from build123d import *

# Parameters (mm, degrees)
SKETCH1_R           = 29.5
BOSS_EXTRUDE1_DEPTH = 6
SKETCH2_R           = 15
BOSS_EXTRUDE2_DEPTH = 25
SKETCH3_R           = 3
CUT_EXTRUDE1_DEPTH  = 25
SKETCH4_R           = 2.5
CUT_EXTRUDE2_DEPTH  = 25


with BuildPart() as part:
    # Sketch1 → Boss-Extrude1 (new body)
    with BuildSketch(Plane(origin=(0, 0, 0), x_dir=(0, 0, -1), z_dir=(1, 0, 0))):
        Circle(SKETCH1_R)
    extrude(amount=BOSS_EXTRUDE1_DEPTH)

    # Sketch2 → Boss-Extrude2 (add)
    with BuildSketch(Plane(origin=(6, 0, 0), x_dir=(0, 0, -1), z_dir=(1, 0, 0))):
        Circle(SKETCH2_R)
    extrude(amount=BOSS_EXTRUDE2_DEPTH)

    # Sketch3 → Cut-Extrude1 (cut)
    with BuildSketch(Plane(origin=(31, 0, 0), x_dir=(0, 0, -1), z_dir=(1, 0, 0))):
        Circle(SKETCH3_R)
    extrude(amount=-CUT_EXTRUDE1_DEPTH, mode=Mode.SUBTRACT)

    # Sketch4 → Cut-Extrude2 (cut)
    with BuildSketch(Plane(origin=(6, 0, 0), x_dir=(0, 0, -1), z_dir=(1, 0, 0))):
        with Locations((0, 23.75)):
            Circle(SKETCH4_R)
        with Locations((20.56810334, 11.875)):
            Circle(SKETCH4_R)
        with Locations((20.56810334, -11.875)):
            Circle(SKETCH4_R)
        with Locations((0, -23.75)):
            Circle(SKETCH4_R)
        with Locations((-20.56810334, -11.875)):
            Circle(SKETCH4_R)
        with Locations((-20.56810334, 11.875)):
            Circle(SKETCH4_R)
    extrude(amount=-CUT_EXTRUDE2_DEPTH, mode=Mode.SUBTRACT)


solid = part.part
Geometry: final body of the model. Coordinates: model frame, mm. A direction names the side the tool comes from. Round coordinates to 2 decimals unless told otherwise and drop trailing zeros. Loops run counter-clockwise (first coordinate to the right, second up) from the corner with the lowest first, then second, coordinate; pieces in that order, holes last. Notation, with made-up numbers: M 8,10.5 L 29,10.5 A20 cw 29,19.5 Z; hole C -6.75,38 d2. An arc over 180 degrees is marked long. Put each result on its own line as item: value. Start each with the question number.
(1) Section query D-D (y = -23.75). Return loops of the section in (x, z), then the cut area to 3 significant figures.
(2) Section query B-B (y = 0). Return loops of the section in (x, z), then the cut area to 3 significant figures.
(3) Section query C-C (y = 13). Return loops of the section in (x, z).
(4) Set-up query: faces 5 (the face through (6, 0, 0)), 6 (the face through (3.04, 26.23, 0.33)). Return all of +Z, -Z, +X, -X, +Y, -Y with unobstructed straight access to the full face (end or side cutting, diameter ignored); none if empty.
(5) Contact query for flat-ended pins moving along their axis: pin 1 Ø5 at (x, z) = (26.5, -4) entering from -Y; pin 2 Ø5 at (x, z) = (25, 2.5) entering from -Y; pin 3 Ø8 at (y, z) = (11.88, -20.57) entering from +X. Output: stop coordinate, or through.
(6) Draft query along Y for faces 1 (the face through (0, 0, 0)), 2 (the face through (18.325, 0.66, 14.985)), 3 (the face through (19, 0, 3)), 4 (the face through (3.04, -13.4, 22.55)). Return one class per face: +Y half, -Y half, draft (parallel to the pull), parting line (faces both ways), or undercut.
(7) Section query A-A (z = 0). Return loops of the section in (x, y), then the cut area to 3 significant figures.
(8) Material intervals for line 1 along Y through (x, z) = (11, 0); line 2 along X through (y, z) = (-24.5, 4); line 3 along Y through (x, z) = (24, 2.5), sorted ascending. Write a range as [from, to].
Findings below:
1. outline: M 0,-17.5 L 6,-17.5 L 6,-2.5 L 0,-2.5 Z; M 0,2.5 L 6,2.5 L 6,17.5 L 0,17.5 Z
1. area: 180 mm2
2. outline: M 0,-29.5 L 6,-29.5 L 6,-15 L 31,-15 L 31,-3 L 6,-3 L 6,3 L 31,3 L 31,15 L 6,15 L 6,29.5 L 0,29.5 Z
2. area: 954 mm2
3. outline: M 0,-26.48 L 6,-26.48 L 6,-22.8 L 0,-22.8 Z; M 0,-18.34 L 6,-18.34 L 6,-7.48 L 31,-7.48 L 31,7.48 L 6,7.48 L 6,18.34 L 0,18.34 Z; M 0,22.8 L 6,22.8 L 6,26.48 L 0,26.48 Z
4. face 5: +X
4. face 6: +X, -X
5. pin 1: stops at y = -14.92
5. pin 2: stops at y = -15
5. pin 3: stops at x = 6
6. face 1: draft
6. face 2: parting line
6. face 3: undercut
6. face 4: undercut
7. outline: M 0,-29.5 L 6,-29.5 L 6,-26.25 L 0,-26.25 Z; M 0,-21.25 L 6,-21.25 L 6,-15 L 31,-15 L 31,-3 L 6,-3 L 6,3 L 31,3 L 31,15 L 6,15 L 6,21.25 L 0,21.25 Z; M 0,26.25 L 6,26.25 L 6,29.5 L 0,29.5 Z
7. area: 894 mm2
8. line 1: y = [-15, -3], [3, 15]
8. line 2: x = [0, 6]
8. line 3: y = [-14.79, -1.66], [1.66, 14.79]
